from build123d import *

# Parameters (mm, degrees)
CUT_EXTRUDE1_DEPTH = 1.2
FILLET1_R          = 0.15


with BuildPart() as part:
    # Sketch1 → Revolve1 (revolve)
    with BuildSketch(Plane.XY, mode=Mode.PRIVATE) as revolve1_sk:
        Polygon((0, 0), (0, 1.5), (7.5, 1.5), (8, 1), (8, 0), align=None)
    revolve(revolve1_sk.sketch.rotate(Axis((8, 0, 0), (-1, 0, 0)), 90), axis=Axis((8, 0, 0), (-1, 0, 0)))

    # Sketch2 → Cut-Extrude1 (cut)
    with BuildSketch(Plane.ZY):
        Polygon((0.433012702, 0.75), (-0.433012702, 0.75), (-0.866025404, 0), (-0.433012702, -0.75), (0.433012702, -0.75), (0.866025404, 0), align=None)
    extrude(amount=-CUT_EXTRUDE1_DEPTH, mode=Mode.SUBTRACT)

    # Fillet1
    fillet1_edges = [part.edges().sort_by_distance(p)[0] for p in [
        (0, 0, 1.5),
    ]]
    fillet(fillet1_edges, radius=FILLET1_R)


solid = part.part
Part model, mm, in its own coordinate system. A direction names the side the tool comes from. Give positions to 0.01 mm unless a question says otherwise; leave off trailing zeros. Loops run counter-clockwise (first coordinate to the right, second up) from the corner with the lowest first, then second, coordinate; pieces in that order, holes last. Notation, with made-up numbers: (73.5, 16.5) -> (94.5, 16.5) arc R37 ccw to (94.5, 52.5) -> close; hole circle Ø3 at (-28, 70). An arc over 180 degrees is marked (long way). Write each question's results on one line, items separated by ' | '. Start each with the question number.
Q1. Which spindle directions (+Z, -Z, +X, -X, +Y, -Y) get a long thin tool onto all of the face, cutting with end or side? Do faces 1 (the face through (1.2, 0, 0)), 2 (the face through (0, 1, 0)). Say none if no direction does.
Q2. Wall check: L1, parallel to X at y = -0.45, z = 0.2; L2, parallel to Z at x = 0.5, y = 0.45; L3, parallel to X at y = 0.15, z = -1.15. Give the ranges that are in metal, low to high.
Q3. Band-saw the part on B-B on z = 0. List the corners of the cut face in (x, y).
Q4. Band-saw the part on C-C on x = 5.5. List the corners of the cut face in (y, z).
Q5. Pin check, flat tips, straight feed: P1, Ø0.5, axis at y = 0, z = 0, coming from the -X side; P2, Ø1.5, axis at x = 4, y = -0.5, coming from the +Z side; P3, Ø1, axis at x = 4.5, y = 1, coming from the -Z side. Stop position of each tip, or through.
Q6. Band-saw the part on A-A on x = 1. List the corners of the cut face in (y, z), plus the area to 3 significant figures.
Q7. Pull direction Z, two halves, no side cores. Call faces 3 (the face through (3.88, -0.45, -1.43)), 4 (the face through (1, -0.75, 0)), 5 (the face through (8, 0, 0)): +Z half, -Z half, draft (parallel to the pull), parting line (faces both ways), or undercut.
Results are:
1) face 1: -X | face 2: +Z, -Z, -X, +Y, -Y
2) L1: x = 1.2 to 8 | L2: z = -1.43 to -0.61, 0.61 to 1.43 | L3: x = 0 to 7.84
3) outline: (0, -1.35) arc R0.15 ccw to (0.15, -1.5) -> (7.5, -1.5) -> (8, -1) -> (8, 1) -> (7.5, 1.5) -> (0.15, 1.5) arc R0.15 ccw to (0, 1.35) -> (0, 0.75) -> (1.2, 0.75) -> (1.2, -0.75) -> (0, -0.75) -> close
4) outline: circle Ø3 at (0, 0)
5) P1: stops at x = 1.2 | P2: stops at z = 1.5 | P3: stops at z = -1.41
6) outline: circle Ø3 at (0, 0); hole (-0.75, -0.43) -> (0, -0.87) -> (0.75, -0.43) -> (0.75, 0.43) -> (0, 0.87) -> (-0.75, 0.43) -> close | area: 5.12 mm²
7) face 3: parting line | face 4: undercut | face 5: draft
